Geometry: final body of the model. Coordinates: model frame, mm. Face numbers are marked on the shaded views. A direction names the side the tool comes from. Round coordinates to 2 decimals unless told otherwise and drop trailing zeros. Loops run counter-clockwise (first coordinate to the right, second up) from the corner with the lowest first, then second, coordinate; pieces in that order, holes last. Notation, with made-up numbers: (12.5, 74) - (23.5, 74) arc R28 ccw to (23.5, 113) - close; hole circle Ø9 at (74, 76.25). An arc over 180 degrees is marked (long way). Answer as a JSON object with one key per item and string values. Group by question number.
Item 1: Section B-B (z = 15). Return the cut outline in (x, y).
Item 2: Line query: line 1 (Y direction, x = -9.75, z = 15); line 2 (Y direction, x = -18.7, z = 15); line 3 (Z direction, x = -7, y = 37.5). Output: solid intervals per line, ascending.
Item 3: First-contact query: pin 1 (6 mm diameter, centred on x = -16.5, z = 1, fed in from +Y); pin 2 (4 mm diameter, centred on y = 40.5, z = 21, fed in from +X); pin 3 (2 mm diameter, centred on x = -8.5, z = 21, fed in from +Y). Flat tips, straight axial feed; report the tip coordinate or a pass-through.
Item 4: Draft query along Y for the marked faces 4, 5 and 6. Return one class per face: released by +Y, released by -Y, zero draft, split by the parting line, or undercut.
Item 5: Reachability of the marked faces 1, 2 and 3 from +Z, -Z, +X, -X, +Y, -Y: full face, straight path, thin tool, end or side. Return the list, or none.
Item 6: Section A-A (x = -11.5). Return the cut outline in (y, z), plus the area to 3 significant figures.
Item 7: Section D-D (x = -16.25). Return the cut outline in (y, z), plus the area to 3 significant figures.
Item 8: Section C-C (y = 35). Return the cut outline in (x, z).
```python
from build123d import *

# Parameters (mm, degrees)
SALIENTE_EXTRUIR1_DEPTH = 20
CROQUIS5_R              = 17.5
CORTAR_EXTRUIR1_DEPTH   = 15
CROQUIS6_R              = 4
CROQUIS6_R_2            = 1.5
CORTAR_EXTRUIR2_DEPTH   = 6
CROQUIS7_R              = 3
CORTAR_EXTRUIR3_DEPTH   = 2


with BuildPart() as part:
    # Croquis3 → Saliente-Extruir1 (new body)
    with BuildSketch(Plane(origin=(0, 0, 0), x_dir=(0, 0, -1), z_dir=(1, 0, 0))):
        with BuildLine():
            Line((27.255557931, 9.68339194), (10.161648688, 38.854157713))
            ThreePointArc((10.161648688, 38.854157713), (9.28194474, 40.533010779), (8.565114788, 42.287599469))
            ThreePointArc((8.565114788, 42.287599469), (-27.147634239, 55.790109054), (-34.527859081, 18.330123878))
            ThreePointArc((-34.527859081, 18.330123878), (-31.582921761, 13.275948256), (-30.226287359, 7.585878825))
            Line((-30.226287359, 7.585878825), (-30.076141014, 5.870094713))
            ThreePointArc((-30.076141014, 5.870094713), (-30.019044321, 4.999168316), (-30, 4.126580134))
            Line((-30, 4.126580134), (-30, -5))
            Line((-30, -5), (30, -5))
            Line((30, -5), (30, -0.428270658))
            ThreePointArc((30, -0.428270658), (29.301698871, 4.810471624), (27.255557931, 9.68339194))
        make_face()
    extrude(amount=-SALIENTE_EXTRUIR1_DEPTH)

    # Croquis5 → Cortar-Extruir1 (cut)
    with BuildSketch(Plane(origin=(0, 0, 0), x_dir=(0, 0, -1), z_dir=(1, 0, 0))):
        with Locations((-15, 35)):
            Circle(CROQUIS5_R)
    extrude(amount=-CORTAR_EXTRUIR1_DEPTH, mode=Mode.SUBTRACT)

    # Croquis6 → Cortar-Extruir2 (cut)
    with BuildSketch(Plane(origin=(-15, 0, 0), x_dir=(0, 0, -1), z_dir=(1, 0, 0))):
        with Locations((-15, 35)):
            Circle(CROQUIS6_R)
        with Locations((-6.25, 35)):
            Circle(CROQUIS6_R_2)
        with Locations((-23.75, 35)):
            Circle(CROQUIS6_R_2)
    extrude(amount=-CORTAR_EXTRUIR2_DEPTH, mode=Mode.SUBTRACT)

    # Croquis7 → Cortar-Extruir3 (cut)
    with BuildSketch(Plane.ZY.offset(20)):
        with Locations((6.25, 35)):
            Circle(CROQUIS7_R)
        with Locations((23.75, 35)):
            Circle(CROQUIS7_R)
    extrude(amount=-CORTAR_EXTRUIR3_DEPTH, mode=Mode.SUBTRACT)


solid = part.part
```
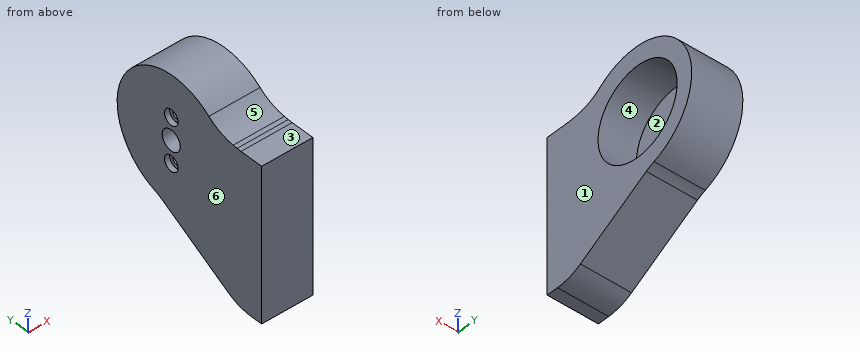
Values:
{
 "1": {"outline": "(-20, -5) - (0, -5) - (0, 17.5) - (-15, 17.5) - (-15, 31) - (-20, 31) - close; (-20, 39) - (-15, 39) - (-15, 52.5) - (0, 52.5) - (0, 58.94) - (-20, 58.94) - close"},
 "2": {"line 1": "y = -5 to 17.5, 52.5 to 58.94", "line 2": "y = -5 to 31, 39 to 58.94", "line 3": "z = -10.96 to -2.32, 32.32 to 39.75"},
 "3": {"pin 1": "stops at y = 56.39", "pin 2": "stops at x = -15", "pin 3": "stops at y = 58.43"},
 "4": {"face 4": "undercut", "face 5": "released by -Y", "face 6": "zero draft"},
 "5": {"face 1": "+Z, -Z, +X, +Y, -Y", "face 2": "+X", "face 3": "+Z, +X, -X, -Y"},
 "6": {"outline": "(-5, -30) - (-0.43, -30) arc R20 ccw to (9.68, -27.26) - (38.85, -10.16) arc R20 cw to (42.29, -8.57) arc R25 ccw (long way) to (18.33, 34.53) arc R20 cw to (7.59, 30.23) - (5.87, 30.08) arc R20 cw to (4.13, 30) - (-5, 30) - close; hole circle Ø35 at (35, 15)", "area": "2,270 mm^2"},
 "7": {"outline": "(-5, -30) - (-0.43, -30) arc R20 ccw to (9.68, -27.26) - (38.85, -10.16) arc R20 cw to (42.29, -8.57) arc R25 ccw (long way) to (18.33, 34.53) arc R20 cw to (7.59, 30.23) - (5.87, 30.08) arc R20 cw to (4.13, 30) - (-5, 30) - close; hole circle Ø8 at (35, 15); hole circle Ø3 at (35, 6.25); hole circle Ø3 at (35, 23.75)", "area": "3,160 mm^2"},
 "8": {"outline": "(-20, -12.42) - (0, -12.42) - (0, -2.5) - (-15, -2.5) - (-15, 4.75) - (-18, 4.75) - (-18, 3.25) - (-20, 3.25) - close; (-20, 9.25) - (-18, 9.25) - (-18, 7.75) - (-15, 7.75) - (-15, 11) - (-20, 11) - close; (-20, 19) - (-15, 19) - (-15, 22.25) - (-18, 22.25) - (-18, 20.75) - (-20, 20.75) - close; (-20, 26.75) - (-18, 26.75) - (-18, 25.25) - (-15, 25.25) - (-15, 32.5) - (0, 32.5) - (0, 39.98) - (-20, 39.98) - close"}
}
